```python
from build123d import *

# Parameters (mm, degrees)
SKETCH1_W                    = 38.1
SKETCH1_H                    = 38.1
MAIN_BODY_DEPTH              = 34
F_9_32_RIGHT_RAIL_DEPTH      = 64.712008287
F_9_32_RIGHT_RAIL_DEPTH_BACK = 5.55625
SKETCH3_R                    = 3.571875
SKETCH4_R                    = 3.571875
F_9_32_LEFT_RAIL_DEPTH       = 5.55625
F_9_32_TOPPER_DEPTH          = 64.712008287
F_9_32_TOPPER_DEPTH_BACK     = 10
SKETCH8_R                    = 3.571875
CUT_EXTRUDE3_START           = -5.55625
CUT_EXTRUDE3_DEPTH           = 32.54375
CUT_EXTRUDE4_START           = -5.55625
CUT_EXTRUDE4_DEPTH           = 32.54375
CUT_EXTRUDE12_START          = -30.825
CUT_EXTRUDE12_OUTLINE_W      = 29.119345377
CUT_EXTRUDE12_OUTLINE_H      = 29.119345377
CUT_EXTRUDE12_DEPTH          = 22.09375
CUT_EXTRUDE15_START          = -17
CUT_EXTRUDE15_DEPTH          = 13.825
CUT_EXTRUDE16_REACH          = 65.712
CUT_EXTRUDE17_REACH          = 65.712


# Read off the part's stored shape, not the designer's step: Cut-Extrude12
with BuildPart() as part:
    # Sketch1 → Main Body (new body)
    with BuildSketch(Plane(origin=(0, 0, 0), x_dir=(1, 0, 0), z_dir=(0, 1, 0))):
        with Locations((19.05, 19.05)):
            Rectangle(SKETCH1_W, SKETCH1_H)
    extrude(amount=MAIN_BODY_DEPTH)

    # Sketch3 → 9/32 Right Rail (cut, two sides: drawn at the far end of the back side and taken through both)
    with BuildSketch(Plane.XY.offset(-F_9_32_RIGHT_RAIL_DEPTH_BACK)):
        with Locations(Location((19.05, 17, 0), (0, 0, 180))):
            Circle(SKETCH3_R)
    extrude(amount=F_9_32_RIGHT_RAIL_DEPTH + F_9_32_RIGHT_RAIL_DEPTH_BACK, mode=Mode.SUBTRACT)

    # Sketch4 → 9/32 Left Rail (cut)
    with BuildSketch(Plane.ZY):
        with Locations((-19.05, 17)):
            Circle(SKETCH4_R)
    extrude(amount=-F_9_32_LEFT_RAIL_DEPTH, mode=Mode.SUBTRACT)

    # Sketch8 → 9/32 Topper (cut, two sides: drawn at the far end of the back side and taken through both)
    with BuildSketch(Plane(origin=(0, 34, 0), x_dir=(1, 0, 0), z_dir=(0, 1, 0)).offset(-F_9_32_TOPPER_DEPTH_BACK)):
        with Locations(Location((19.05, 19.05, 0), (0, 0, 90))):
            Circle(SKETCH8_R)
    extrude(amount=F_9_32_TOPPER_DEPTH + F_9_32_TOPPER_DEPTH_BACK, mode=Mode.SUBTRACT)

    # Sketch9 → Cut-Extrude3 (cut)
    with BuildSketch(Plane.ZY.offset(CUT_EXTRUDE3_START)):
        Polygon((-22.372470377, 22.7546875), (-25.694940754, 17), (-22.372470377, 11.2453125), (-15.727529623, 11.2453125), (-12.405059246, 17), (-15.727529623, 22.7546875), align=None)
    extrude(amount=-CUT_EXTRUDE3_DEPTH, mode=Mode.SUBTRACT)

    # Sketch10 → Cut-Extrude4 (cut)
    with BuildSketch(Plane.XY.offset(CUT_EXTRUDE4_START)):
        Polygon((15.727529623, 22.7546875), (12.405059246, 17), (15.727529623, 11.2453125), (22.372470377, 11.2453125), (25.694940754, 17), (22.372470377, 22.7546875), align=None)
    extrude(amount=-CUT_EXTRUDE4_DEPTH, mode=Mode.SUBTRACT)

    # Cut-Extrude12 outline → Cut-Extrude12 (cut)
    with BuildSketch(Plane(origin=(0, 34, 0), x_dir=(1, 0, 0), z_dir=(0, 1, 0)).offset(CUT_EXTRUDE12_START)):
        with Locations((23.540327312, 23.540327312)):
            Rectangle(CUT_EXTRUDE12_OUTLINE_W, CUT_EXTRUDE12_OUTLINE_H)
    extrude(amount=CUT_EXTRUDE12_DEPTH, mode=Mode.SUBTRACT)

    # Sketch14 → Cut-Extrude15 (cut)
    with BuildSketch(Plane(origin=(0, 34, 0), x_dir=(1, 0, 0), z_dir=(0, 1, 0)).offset(CUT_EXTRUDE15_START)):
        Polygon((23.748682668, 14.351317332), (25.468519889, 20.769837221), (20.769837221, 25.468519889), (14.351317332, 23.748682668), (12.631480111, 17.330162779), (17.330162779, 12.631480111), align=None)
    extrude(amount=CUT_EXTRUDE15_DEPTH, mode=Mode.SUBTRACT)

    # Sketch15 → Cut-Extrude16 (cut, up to next)
    with BuildSketch(Plane.XZ, mode=Mode.PRIVATE) as cut_extrude16_sk1:
        Polygon((38.1, -8.980654623), (8.980654623, -38.1), (38.1, -38.1), align=None)
    cut_extrude16_tool1 = extrude(cut_extrude16_sk1.sketch, amount=-CUT_EXTRUDE16_REACH, mode=Mode.PRIVATE) & part.part
    add(cut_extrude16_tool1.solids().sort_by_distance((28.393552, 0, -28.393552))[0], mode=Mode.SUBTRACT)

    # Sketch16 → Cut-Extrude17 (cut, up to next)
    with BuildSketch(Plane(origin=(0, 34, 0), x_dir=(1, 0, 0), z_dir=(0, 1, 0)), mode=Mode.PRIVATE) as cut_extrude17_sk1:
        Polygon((38.1, 38.1), (16.276714219, 38.1), (38.1, 16.276714219), align=None)
    cut_extrude17_tool1 = extrude(cut_extrude17_sk1.sketch, amount=-CUT_EXTRUDE17_REACH, mode=Mode.PRIVATE) & part.part
    add(cut_extrude17_tool1.solids().sort_by_distance((30.825571, 34, -30.825571))[0], mode=Mode.SUBTRACT)


solid = part.part
```
Verification items for the finished model (mm, model axes). A direction names the side the tool comes from. Coordinates: 2 decimals unless noted, no trailing zeros. Loops run counter-clockwise (first coordinate to the right, second up) from the corner with the lowest first, then second, coordinate; pieces in that order, holes last. Notation, with made-up numbers: (-35, 39.25) -> (17, 39.25) arc R14 cw to (17, 62.25) -> close; hole circle Ø9 at (15, 48). An arc over 180 degrees is marked (long way). Put each result on its own line as item: value.
1. Tool access check on faces 1 (the face through (19, 22.755, -7)), 2 (the face through (23.15, 28.01, -23.09)), 3 (the face through (8.981, 12, -23)). Record the directions out of +Z, -Z, +X, -X, +Y, -Y that give a thin tool (end or side, any length) a straight path to the whole face; none if there is none.
Result set:
face 1: -Z
face 2: none
face 3: -Z, +X
2. Section check D-D, the plane x = 19.05. Record the boundary of the cut face in (y, z) (3 decimals), then the cut area to 3 significant figures.
Result set:
outline: (0, -28.031) -> (3.175, -28.031) -> (3.175, -8.981) -> (11.245, -8.981) -> (11.245, -5.556) -> (13.428, -5.556) -> (13.428, 0) -> (0, 0) -> close; (20.572, -5.556) -> (22.755, -5.556) -> (22.755, -8.981) -> (25.269, -8.981) -> (25.269, -13.092) -> (30.825, -13.092) -> (30.825, -15.478) -> (34, -15.478) -> (34, 0) -> (20.572, 0) -> close; (25.269, -35.327) -> (34, -35.327) -> (34, -22.622) -> (30.825, -22.622) -> (30.825, -25.008) -> (25.269, -25.008) -> close
area: 428 mm^2
3. Section check B-B, the plane x = 8. Record the boundary of the cut face in (y, z).
Result set:
outline: (0, -38.1) -> (34, -38.1) -> (34, 0) -> (0, 0) -> close; hole (11.25, -22.37) -> (17, -25.69) -> (22.75, -22.37) -> (22.75, -15.73) -> (17, -12.41) -> (11.25, -15.73) -> close
4. Section check C-C, the plane z = -4. Record the boundary of the cut face in (x, y).
Result set:
outline: (0, 0) -> (38.1, 0) -> (38.1, 34) -> (0, 34) -> close; hole circle Ø7.14 at (19.05, 17)
5. Thickness scan on line 1 (Y direction, x = 19, z = -1); line 2 (Y direction, x = 11, z = -31) (3 decimals); line 3 (Z direction, x = 20, y = 10). Record the ranges inside material, lowest first.
Result set:
line 1: y = 0 to 13.43, 20.57 to 34
line 2: y = 0 to 3.175, 25.269 to 34
line 3: z = -8.98 to 0
6. Mould release check, pull along Z, two halves, no side actions. Record for faces 4 (the face through (27.036, 29.695, -27.341)), 5 (the face through (22.537, 32.39, -18.276)), 6 (the face through (0, 13, -19)): pulls with the +Z half, pulls with the -Z half, needs draft (parallel to the pull), parting line crosses it, or undercut.
Result set:
face 4: pulls with the -Z half
face 5: undercut
face 6: needs draft
7. Gauge pin test, flat ends, axial feed: P1, Ø8, axis at x = 11, z = -4.5, coming from the -Y side; P2, Ø4, axis at y = 20.5, z = -31.5, coming from the +X side; P3, Ø12.5, axis at x = 21.5, y = 16.5, coming from the -Z side; P4, Ø2, axis at y = 15.5, z = -22.5, coming from the +X side. Record the tip position at first contact, or that the pin passes through.
Result set:
P1: stops at y = 0
P2: stops at x = 8.98
P3: stops at z = -8.98
P4: stops at x = 5.56
8. Section check A-A, the plane y = 14. Record the boundary of the cut face in (x, z).
Result set:
outline: (0, -38.1) -> (8.98, -38.1) -> (8.98, -23.96) -> (5.56, -23.96) -> (5.56, -20.99) -> (0, -20.99) -> close; (0, -17.11) -> (5.56, -17.11) -> (5.56, -14.14) -> (8.98, -14.14) -> (8.98, -8.98) -> (14.14, -8.98) -> (14.14, -5.56) -> (17.11, -5.56) -> (17.11, 0) -> (0, 0) -> close; (20.99, -5.56) -> (23.96, -5.56) -> (23.96, -8.98) -> (38.1, -8.98) -> (38.1, 0) -> (20.99, 0) -> close
